Here's how the part is built. I have some questions about the finished solid (model axes, mm). A direction names the side the tool comes from. Coordinates: 2 decimals unless noted, no trailing zeros. Loops run counter-clockwise (first coordinate to the right, second up) from the corner with the lowest first, then second, coordinate; pieces in that order, holes last. Notation, with made-up numbers: (8, -2) -> (65, -2) arc R12 cw to (65, 11) -> close; hole circle Ø6 at (-8.75, 64). An arc over 180 degrees is marked (long way). Answer as a JSON object with one key per item and string values. Group by question number.
1) I want a section at C-C (y = 9). Write out the boundary of the cut face in (x, z), then the cut area to 3 significant figures.
2) I need wall thicknesses on probe 1 along Z at (x, y) = (7.5, -4.25); probe 2 along X at (y, z) = (10, 5.5); probe 3 along X at (y, z) = (3.25, 3). Which ranges of each line are inside material? Lowest first, please. Write a range as [from, to].
3) I want a section at A-A (z = 0). Write out the boundary of the cut face in (x, y).
4) I want a section at B-B (x = 4). Write out the boundary of the cut face in (y, z), then the cut area to 3 significant figures.
5) Which directions (+Z, -Z, +X, -X, +Y, -Y) give clear straight access to the entire face, cutting with the end or side of a thin tool? Please do faces 1 (the flat face through (-2, 0, 5)), 2 (the cylindrical face through (27, -6, 0)), 3 (the conical face through (-4.7, -5.17, 0.11)), 4 (the flat face through (-22.5, 0, 0)), 5 (the flat face through (-2, 0, -5)).
6) I'm going to push flat-ended pins straight in: pin 1 (2 mm diameter, centred on x = 30, y = -6.5, fed in from +Z); pin 2 (1.1 mm diameter, centred on y = 0, z = -5.5, fed in from -X); pin 3 (2 mm diameter, centred on x = 52.5, y = -4.5, fed in from -Z). Where does each tip first touch, or does it pass through?
7) I want a section at D-D (z = 7.5). Write out the boundary of the cut face in (x, y).
Autodesk Inventor part; units mm, degrees
ref_plane "ROD_BODY_XY" through (0, 0, 0) normal (1, 0, 0) x (0, 0, -1)
ref_plane "ROD_BODY_YZ" through (0, 0, 0) normal (0, 0, -1) x (0, 1, 0)
ref_plane "ROD_BODY_ZX" through (0, 0, 0) normal (0, 1, 0) x (1, 0, 0)
sketch "Sketch_3" plane through (0, 0, 0) normal (0, 0, 1) x (1, 0, 0)
  line L0 (61.25, 0) -> (-22.5, 0)
  line L1 (-22.5, 0) -> (-22.5, 4.233)
  line L2 (-22.5, 4.233) -> (-21.733, 5)
  line L3 (-21.733, 5) -> (-5, 5)
  line L4 (-5, 5) -> (-3.2679, 6)
  line L5 (-3.2679, 6) -> (56.25, 6)
  line L6 (56.25, 6) -> (56.25, 12.5)
  line L7 (56.25, 12.5) -> (61.25, 12.5)
  line L8 (61.25, 12.5) -> (61.25, 0)
  line L9 (61.25, 0) -> (-22.5, 0)
revolve "Revolution1" add sketch "Sketch_3" angle 360 about axis through (61.25, 0, 0) along (1, 0, 0)
thread "Thread1"
sketch "Sketch_7" plane through (0, 0, 0) normal (1, 0, 0) x (0, 0, -1)
  circle A0 centre (0, 0) radius 12
  line L0 (-5, 7) -> (-5, -7)
  line L1 (-5, -7) -> (5, -7)
  line L2 (5, -7) -> (5, 7)
  line L3 (5, 7) -> (-5, 7)
extrude "Extrusion1" cut sketch "Sketch_7" against normal blind 5
ref_plane "ROD_BODY_XY" through (0, 0, 0) normal (1, 0, 0) x (0, 0, -1)
ref_plane "ROD_BODY_YZ" through (0, 0, 0) normal (0, 0, -1) x (0, 1, 0)
ref_plane "ROD_BODY_ZX" through (0, 0, 0) normal (0, 1, 0) x (1, 0, 0)
ref_plane "ROD_NUT_XY" through (-22.5, 0, 0) normal (-1, 0, 0) x (0, 0, -1)
ref_plane "ROD_NUT_YZ" through (-22.5, 0, 0) normal (0, 0, -1) x (0, -1, 0)
ref_plane "ROD_NUT_ZX" through (-22.5, 0, 0) normal (0, -1, 0) x (-1, 0, 0)
properties part number "CDQSB25-40DM(1_0)_ROD"
Determined:
{
 "1": {"outline": "(56.25, -8.67) -> (61.25, -8.67) -> (61.25, 8.67) -> (56.25, 8.67) -> close", "area": "86.7 mm^2"},
 "2": {"probe 1": "[-4.24, 4.24]", "probe 2": "[56.25, 61.25]", "probe 3": "[-22.31, 61.25]"},
 "3": {"outline": "(-22.5, -4.23) -> (-21.73, -5) -> (-5, -5) -> (-3.27, -6) -> (56.25, -6) -> (56.25, -12.5) -> (61.25, -12.5) -> (61.25, 12.5) -> (56.25, 12.5) -> (56.25, 6) -> (-3.27, 6) -> (-5, 5) -> (-21.73, 5) -> (-22.5, 4.23) -> close"},
 "4": {"outline": "circle Ø12 at (0, 0)", "area": "113 mm^2"},
 "5": {"face 1": "+Z, -X, +Y, -Y", "face 2": "-X", "face 3": "-X, -Y", "face 4": "+Z, -Z, -X, +Y, -Y", "face 5": "-Z, -X, +Y, -Y"},
 "6": {"pin 1": "z = 2.4", "pin 2": "x = -21.78", "pin 3": "z = -4.87"},
 "7": {"outline": "(56.25, -10) -> (61.25, -10) -> (61.25, 10) -> (56.25, 10) -> close"}
}
